For this review, take the finished solid that the model builds, in its own axes (mm). Face numbers are marked on the shaded views. A direction names the side the tool comes from. Give positions to 0.01 mm unless a question says otherwise; leave off trailing zeros. Loops run counter-clockwise (first coordinate to the right, second up) from the corner with the lowest first, then second, coordinate; pieces in that order, holes last. Notation, with made-up numbers: (24, -17) - (64, -17) arc R28 ccw to (64, 11) - close; hole circle Ø4 at (-22, 73.25). An arc over 180 degrees is marked (long way). Put each result on its own line as item: value.
from build123d import *

# Parameters (mm, degrees)
F3_D     = 5.4102
F3_DEPTH = 25.4
F3_TIP   = 1.6253880605
F5_D     = 3.4544
F5_DEPTH = 15.875
F5_TIP   = 1.0378064612
F6_SIZE  = 0.762


with BuildPart() as f1:
    # F0 (on Top) → F1 (revolve)
    with BuildSketch(Plane.XY):
        Polygon((-84.074, 0), (0, 0), (0, 6.35), (-14.224, 6.35), (-14.224, 15.875), (-39.624, 15.875), (-39.624, 9.525), (-84.074, 9.525), align=None)
    revolve(axis=Axis((-42.037, 0, 0), (1, 0, 0)))

    # F3
    with Locations(Plane.YZ):
        with Locations((0, 0)):
            Hole(F3_D / 2, depth=F3_DEPTH)
            with Locations((0, 0, -(F3_DEPTH + F3_TIP / 2))):  # 118° drill point
                Cone(0, F3_D / 2, F3_TIP, mode=Mode.SUBTRACT)

    # F5
    with Locations(Plane.YZ.offset(-14.224)):
        with Locations((-11.1125, 0), (11.1125, 0)):
            Hole(F5_D / 2, depth=F5_DEPTH)
            with Locations((0, 0, -(F5_DEPTH + F5_TIP / 2))):  # 118° drill point
                Cone(0, F5_D / 2, F5_TIP, mode=Mode.SUBTRACT)

    # F6
    f6_edges = [f1.edges().sort_by_distance(p)[0] for p in [
        (0, -6.35, 0),
        (-14.224, -15.875, 0),
        (-39.624, -15.875, 0),
        (-84.074, -9.525, 0),
    ]]
    chamfer(f6_edges, length=F6_SIZE)


solid = f1.part
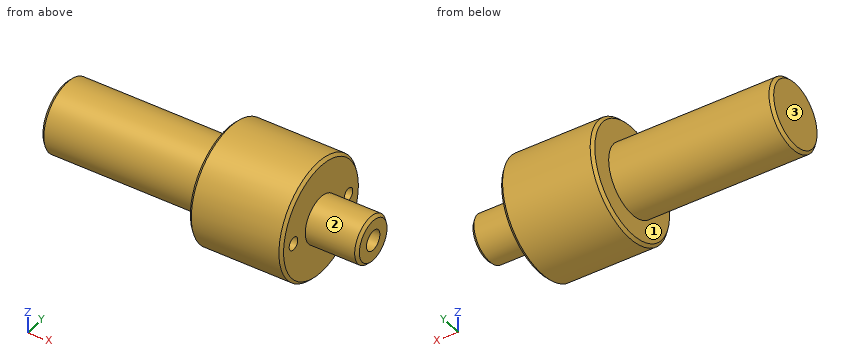
1) Insertion check: pin 1 Ø2 at (x, z) = (-37, 7) entering from -Y; pin 2 Ø3 at (x, y) = (-18, -12.5) entering from +Z; pin 3 Ø7 at (y, z) = (0, 0) entering from +X; pin 4 Ø3 at (y, z) = (-9.5, 1) entering from +X. Each pin has a flat end and moves straight along its axis. Give the tip position at first contact, or say it passes through.
Geometry check:
pin 1: stops at y = -14.7
pin 2: stops at z = 11.45
pin 3: stops at x = 0
pin 4: stops at x = -14.22
2) For the marked faces 1, 2 and 3, list the 3-axis set-ups (+Z, -Z, +X, -X, +Y, -Y) from which the entire face can be reached by the end or side of a thin tool; tool diameter is ignored.
Geometry check:
face 1: -X
face 2: +X
face 3: +Z, -Z, -X, +Y, -Y
3) Wall thickness on line 1 (Z direction, x = -7, y = 0); line 2 (X direction, y = 0, z = -10); line 3 (X direction, y = 3, z = 6.5): over which ranges is each line inside the solid? List them lowest first.
Geometry check:
line 1: z = -6.35 to -2.71, 2.71 to 6.35
line 2: x = -39.62 to -14.22
line 3: x = -84.07 to -14.22
4) Take a section at A-A on x = -44. State the section outline as (y, z) points (3 decimals), and give its area (3 significant figures).
Geometry check:
outline: circle Ø19.05 at (0, 0)
area: 285 mm²
